Source: three-view drawing plus pictorial views. Frame: mm from the lowest corner of the part. Round coordinates to 2 decimals unless told otherwise and drop trailing zeros. Loops run counter-clockwise (first coordinate to the right, second up) from the corner with the lowest first, then second, coordinate; pieces in that order, holes last. Notation, with made-up numbers: M -29,9.25 L -19,9.25 A21 cw -19,37.25 Z; hole C -31.75,-32.5 d8. An arc over 180 degrees is marked long. Write each question's results on one line, items separated by ' | '.
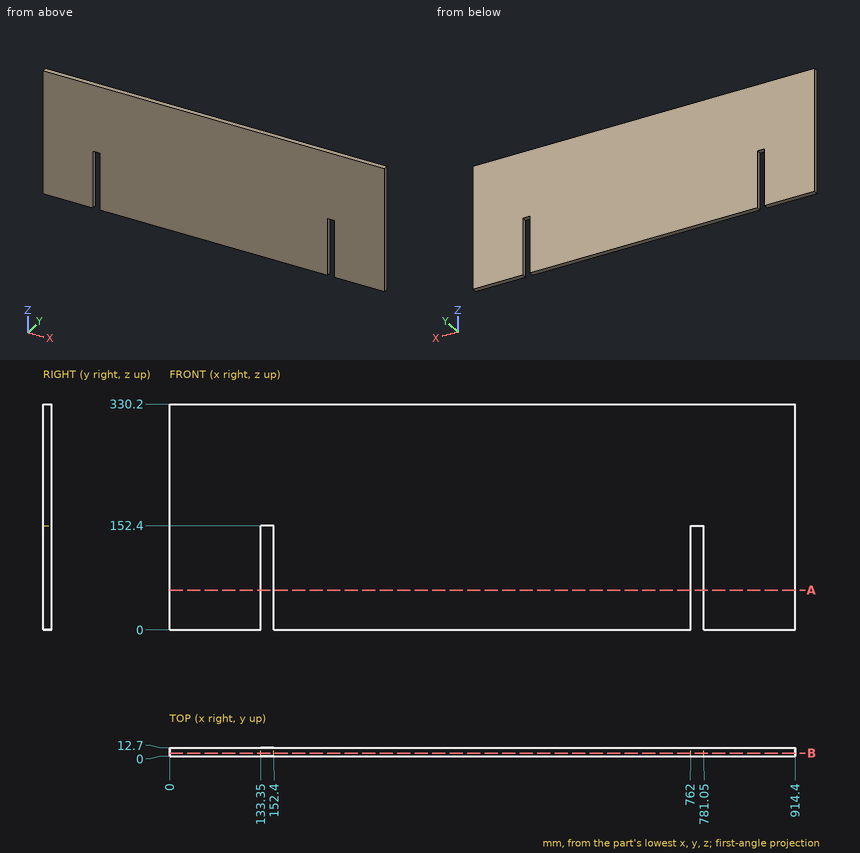
1. Section A-A (z = 58). Output: boundary loops of the cut face in (x, y), then the cut area to 3 significant figures.
Answer key:
outline: M 0,0 L 133.35,0 L 133.35,12.7 L 0,12.7 Z; M 152.4,0 L 762,0 L 762,12.7 L 152.4,12.7 Z; M 781.05,0 L 914.4,0 L 914.4,12.7 L 781.05,12.7 Z | area: 11,100 mm²
2. Ray query, probe 1 along X at (y, z) = (4, 31). Return the intervals inside material, ascending.
Answer key:
probe 1: x = 0 to 133.35, 152.4 to 762, 781.05 to 914.4
3. Section B-B (y = 5). Output: boundary loops of the cut face in (x, z), then the cut area to 3 significant figures.
Answer key:
outline: M 0,0 L 133.35,0 L 133.35,152.4 L 152.4,152.4 L 152.4,0 L 762,0 L 762,152.4 L 781.05,152.4 L 781.05,0 L 914.4,0 L 914.4,330.2 L 0,330.2 Z | area: 296,000 mm²
4. Pin query (flat end, axial travel): P1, Ø6.5, axis at x = 146.5, y = 5, coming from the -Z side. Return the tip coordinate at first contact, or that it passes through.
Answer key:
P1: stops at z = 152.4
